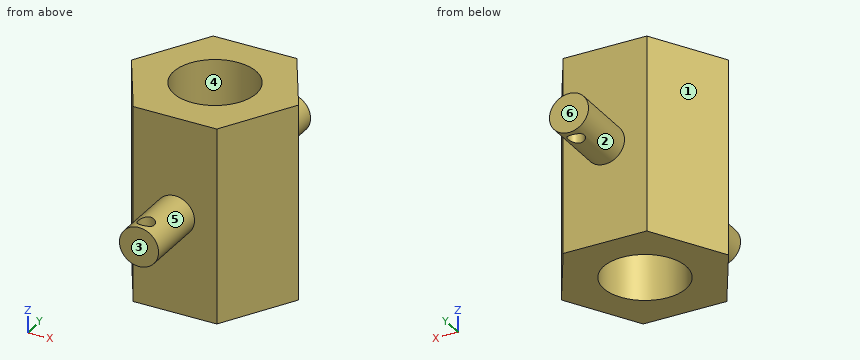
from build123d import *

# Parameters (mm, degrees)
SKETCH1_R           = 6.35
BOSS_EXTRUDE1_DEPTH = 30
SKETCH2_R           = 3
BOSS_EXTRUDE2_DEPTH = 10
SKETCH3_R           = 1.25
CUT_EXTRUDE1_DEPTH  = 39.863708837


with BuildPart() as part:
    # Sketch1 → Boss-Extrude1 (new body)
    with BuildSketch(Plane.XY):
        Polygon((6.415804866, -11.1125), (12.831609733, 0), (6.415804866, 11.1125), (-6.415804866, 11.1125), (-12.831609733, 0), (-6.415804866, -11.1125), align=None)
        Circle(SKETCH1_R, mode=Mode.SUBTRACT)
    extrude(amount=BOSS_EXTRUDE1_DEPTH)

    # Sketch2 → Boss-Extrude2 (add)
    with BuildSketch(Plane.XZ.offset(11.1125)):
        with Locations(Location((0, 15, 0), (0, 0, 180))):
            Circle(SKETCH2_R)
    boss_extrude2 = extrude(amount=BOSS_EXTRUDE2_DEPTH)

    # Sketch3 → Cut-Extrude1 (cut, through all)
    with BuildSketch(Plane.XY):
        with Locations(Location((0, -19.1125, 0), (0, 0, 180))):
            Circle(SKETCH3_R)
    cut_extrude1 = extrude(amount=CUT_EXTRUDE1_DEPTH, mode=Mode.SUBTRACT)

    # Mirror1: Boss-Extrude2, Cut-Extrude1 across plane
    add(boss_extrude2.mirror(Plane.ZX))
    add(cut_extrude1.mirror(Plane.ZX), mode=Mode.SUBTRACT)


solid = part.part
The model under review builds one solid part; all positions refer to its coordinate system, in mm. Face numbers are marked on the shaded views. A direction names the side the tool comes from. Give positions to 0.01 mm unless a question says otherwise; leave off trailing zeros. Write each loop counter-clockwise with the first axis right and the second up, starting at its lowest first coordinate (ties: lowest second). Pieces come first, ordered by that corner, then holes. Notation, with made-up numbers: M -22,-20 L 7,-20 A15 ccw 7,4 Z; hole C 69.5,16 d9. An arc over 180 degrees is marked long. One line per question, with ' | ' between items. Start each with the question number.
Item 1: Wall thickness on line 1 (Y direction, x = 0, z = 15.5); line 2 (Y direction, x = 0, z = 11.25); line 3 (Y direction, x = 2, z = 6.5): over which ranges is each line inside the solid? List them lowest first. Write a range as from..to.
Item 2: We need section C-C on z = 27.75. Write out the cut boundary in (x, y), plus the area to 3 significant figures.
Item 3: We need section B-B on y = -5. Write out the cut boundary in (x, z).
Item 4: For pin 1 (5 mm diameter, centred on y = 15.5, z = 11, fed in from +X); pin 2 (1 mm diameter, centred on x = 3, y = 12.5, fed in from +Z); pin 3 (8 mm diameter, centred on y = 9, z = 13.5, fed in from -X), all flat-tipped, find the tip position at first contact; note any pin that passes through.
Item 5: We need section D-D on x = 4.5. Write out the cut boundary in (y, z).
Item 6: For the marked faces 5 and 6, list the 3-axis set-ups (+Z, -Z, +X, -X, +Y, -Y) from which the entire face can be reached by the end or side of a thin tool; tool diameter is ignored.
Item 7: Draft analysis for pull direction X (two halves, no side actions). For the marked faces 1, 2, 3 and 4, state which applies: released by +X, released by -X, zero draft, split by the parting line, or undercut.
Item 8: We need section A-A on x = 0. Write out the cut boundary in (y, z), plus the area to 3 significant figures.
Results found:
1) line 1: y = -21.11..-20.36, -17.86..-6.35, 6.35..17.86, 20.36..21.11 | line 2: y = -11.11..-6.35, 6.35..11.11 | line 3: y = -11.11..-6.03, 6.03..11.11
2) outline: M -12.83,0 L -6.42,-11.11 L 6.42,-11.11 L 12.83,0 L 6.42,11.11 L -6.42,11.11 Z; hole C 0,0 d12.7 | area: 301 mm2
3) outline: M -9.94,0 L -3.91,0 L -3.91,30 L -9.94,30 Z; M 3.91,0 L 9.94,0 L 9.94,30 L 3.91,30 Z
4) pin 1: stops at x = 2.6 | pin 2: stops at z = 16.66 | pin 3: stops at x = -9.94
5) outline: M -11.11,0 L -4.48,0 L -4.48,30 L -11.11,30 Z; M 4.48,0 L 11.11,0 L 11.11,30 L 4.48,30 Z
6) face 5: -Y | face 6: +Z, -Z, +X, -X, +Y
7) face 1: released by -X | face 2: split by the parting line | face 3: zero draft | face 4: undercut
8) outline: M -21.11,12 L -20.36,12 L -20.36,18 L -21.11,18 Z; M -17.86,12 L -11.11,12 L -11.11,0 L -6.35,0 L -6.35,30 L -11.11,30 L -11.11,18 L -17.86,18 Z; M 6.35,0 L 11.11,0 L 11.11,12 L 17.86,12 L 17.86,18 L 11.11,18 L 11.11,30 L 6.35,30 Z; M 20.36,12 L 21.11,12 L 21.11,18 L 20.36,18 Z | area: 376 mm2
